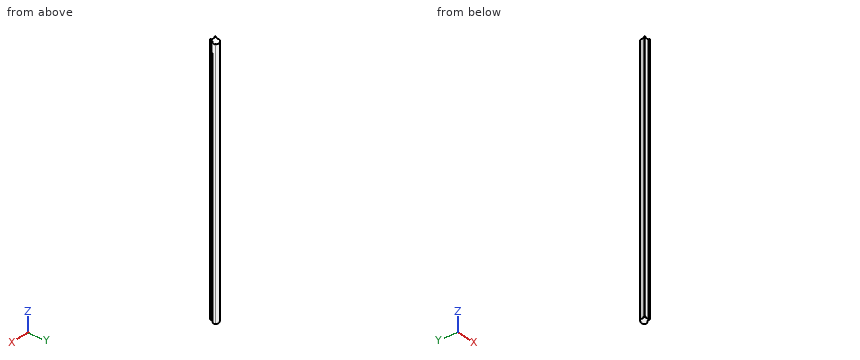
Autodesk Inventor part; units mm, degrees
ref_plane "Конечная плоскость" through (0, 0, 1340.1098) normal (0, 0, 1) x (1, 0, 0)
ref_plane "РабПлоскость4" through (178.641, -785.005, 1769.9053) normal (0, 0.4802388, 0.8771378) x (1, 0, 0)
ref_plane "РабПлоскость5" through (88.641, -691.7426, -766.7409) normal (0, -0.4802388, -0.8771378) x (1, 0, 0)
sketch "Поручень" plane through (0, 0, 0) normal (0, 0, 1) x (1, 0, 0)
  line L0 (20.3655, -7.6059) -> (20.3655, -0.2092)
  line L1 (20.3655, -0.2092) -> (-19.6345, -0.2092)
  line L2 (-19.6345, -0.2092) -> (-19.6345, -7.6059)
  line L3 (-19.6345, -7.6059) -> (-30.865, -7.6059)
  line L4 (-30.865, -7.6059) -> (-30.865, -5.9622)
  line L5 (-30.865, -5.9622) -> (-32.5087, -5.9622)
  line L6 (-32.5087, -5.9622) -> (-32.5087, 0.6126)
  arc A0 (-30.367, 4.2203) -> (-32.5087, 0.6126) centre (-28.3995, 0.6126) ccw
  arc A1 (-30.367, 4.2203) -> (-30.2973, 18.6123) centre (-34.302, 11.4355) ccw
  arc A2 (-24.2902, 41.7054) -> (-30.2973, 18.6123) centre (-24.2902, 29.3776) ccw
  line L7 (-24.2902, 41.7054) -> (-24.2902, 42.9382)
  arc A3 (25.0211, 42.9382) -> (-24.2902, 42.9382) centre (0.3655, 2.9211) ccw
  line L8 (25.0211, 42.9382) -> (25.0211, 41.7054)
  arc A4 (31.0282, 18.6123) -> (25.0211, 41.7054) centre (25.0211, 29.3776) ccw
  arc A5 (31.0282, 18.6123) -> (31.0979, 4.2203) centre (35.033, 11.4355) ccw
  arc A6 (33.2397, 0.6126) -> (31.0979, 4.2203) centre (29.1304, 0.6126) ccw
  line L9 (33.2397, 0.6126) -> (33.2397, -5.9622)
  line L10 (33.2397, -5.9622) -> (31.596, -5.9622)
  line L11 (31.596, -5.9622) -> (31.596, -7.6059)
  line L12 (31.596, -7.6059) -> (20.3655, -7.6059)
  point P0 (0.3655, -0.2092)
  point P1 (0.3655, -7.6059)
sketch "Эскиз" plane through (0, 0, 0) normal (0, 0, 1) x (1, 0, 0)
  line L0 (20, 0) -> (20, 7.3967)
  line L1 (20, 7.3967) -> (-20, 7.3967)
  line L2 (-20, 7.3967) -> (-20, 0)
  line L3 (-20, 0) -> (-31.2305, 0)
  line L4 (-31.2305, 0) -> (-31.2305, 1.6437)
  line L5 (-31.2305, 1.6437) -> (-32.8742, 1.6437)
  line L6 (-32.8742, 1.6437) -> (-32.8742, 8.2186)
  arc A0 (-30.7325, 11.8262) -> (-32.8742, 8.2186) centre (-28.7649, 8.2186) ccw
  arc A1 (-30.7325, 11.8262) -> (-30.6628, 26.2183) centre (-34.6675, 19.0415) ccw
  arc A2 (-24.6557, 49.3113) -> (-30.6628, 26.2183) centre (-24.6557, 36.9835) ccw
  line L7 (-24.6557, 49.3113) -> (-24.6557, 50.5441)
  arc A3 (24.6557, 50.5441) -> (-24.6557, 50.5441) centre (0, 10.527) ccw
  line L8 (24.6557, 50.5441) -> (24.6557, 49.3113)
  arc A4 (30.6628, 26.2183) -> (24.6557, 49.3113) centre (24.6557, 36.9835) ccw
  arc A5 (30.6628, 26.2183) -> (30.7325, 11.8262) centre (34.6675, 19.0415) ccw
  arc A6 (32.8742, 8.2186) -> (30.7325, 11.8262) centre (28.7649, 8.2186) ccw
  line L9 (32.8742, 8.2186) -> (32.8742, 1.6437)
  line L10 (32.8742, 1.6437) -> (31.2305, 1.6437)
  line L11 (31.2305, 1.6437) -> (31.2305, 0)
  line L12 (31.2305, 0) -> (20, 0)
  point P0 (0, 0)
ref_plane "Начальная плоскость" through (0, 0, -1176.9727) normal (0, 0, 1) x (1, 0, 0)
ref_plane "РабПлоскость2" through (0, 0, 1691.8665) normal (0, 0, 1) x (1, 0, 0)
extrude "Тело" add sketch "Эскиз" along normal up to surface (2517.0825 mm away) from surface at -1176.9727
ref_plane "Конечная плоскость" through (0, 0, 1340.1098) normal (0, 0, 1) x (1, 0, 0)
ref_plane "РабПлоскость4" through (178.641, -785.005, 1769.9053) normal (0, 0.4802388, 0.8771378) x (1, 0, 0)
split "Разделение1" plane through (178.641, -785.005, 1769.9053) removes the side toward (0, 0.4802388, 0.8771378)
ref_plane "РабПлоскость5" through (88.641, -691.7426, -766.7409) normal (0, -0.4802388, -0.8771378) x (1, 0, 0)
split "Разделение2" plane through (88.641, -691.7426, -766.7409) removes the side toward (0, -0.4802388, -0.8771378)
equation "\"ШИРИНА\" = 75"
equation "\"ТОЛЩВЫС\" = 58"
equation "\"d0\" = -G_OFFSET_START"
equation "\"СЕЧЕНИЕ_СМЕЩ\" = 0"
equation "\"G_OFFSET_END\" = -351.75672"
equation "\"d4\" = ДЛИНА + G_OFFSET_END"
equation "\"G_OFFSET_START\" = 1176.97268"
equation "\"G_L\" = ДЛИНА + G_OFFSET_START + G_OFFSET_END"
properties part number "Поручень" material "Древесина (дуб)"
CAD build for the part. Positions are in the model's coordinates, mm. Round coordinates to 2 decimals unless told otherwise and drop trailing zeros. Loops run counter-clockwise (first coordinate to the right, second up) from the corner with the lowest first, then second, coordinate; pieces in that order, holes last. Notation, with made-up numbers: M 71,-25 L 78,-25 A18 cw 78,-8 Z; hole C 85,-20 d8. An arc over 180 degrees is marked long. Use a Markdown table: item, result. Add a question column.
(1) Cut at B-B (x = -7). Give the cut face in (y, z), and give its area (3 significant figures).
(2) Cut at A-A (z = 447.5). Give the cut face in (x, y), and give its area (3 significant figures).
(3) Drill centre lines: line 1 (X direction, y = 6.5, z = 1048); line 2 (X direction, y = 40, z = 938); line 3 (Y direction, x = -2.5, z = -538.5). Where is each one in solid material? Low to high.
(4) Flat gauge pins, fed straight in: pin 1 (1.3 mm diameter, centred on y = 0.5, z = -268, fed in from +X); pin 2 (3 mm diameter, centred on x = -26, y = 9.5, fed in from -Z); pin 3 (1.8 mm diameter, centred on y = 0.5, z = -466, fed in from -X); pin 4 (12 mm diameter, centred on y = 35, z = 646, fed in from +X). Where does each tip first touch, or does it go through?
Geometry says:
| question | item | result |
|---|---|---|
| 1 | outline | M 7.4,-1149.52 L 57.01,-1176.69 L 57.01,1308.9 L 7.4,1336.06 Z |
| 1 | area | 123,000 mm² |
| 2 | outline | M -32.87,1.64 L -31.23,1.64 L -31.23,0 L -20,0 L -20,7.4 L 20,7.4 L 20,0 L 31.23,0 L 31.23,1.64 L 32.87,1.64 L 32.87,8.22 A4.11 ccw 30.73,11.83 A8.22 cw 30.66,26.22 A12.33 ccw 24.66,49.31 L 24.66,50.54 A47 ccw -24.66,50.54 L -24.66,49.31 A12.33 ccw -30.66,26.22 A8.22 cw -30.73,11.83 A4.11 ccw -32.87,8.22 Z |
| 2 | area | 3,170 mm² |
| 3 | line 1 | x = -32.87 to -20, 20 to 32.87 |
| 3 | line 2 | x = -36.61 to 36.61 |
| 3 | line 3 | y = 7.4 to 57.46 |
| 4 | pin 1 | stops at x = 31.23 |
| 4 | pin 2 | stops at z = -1151.5 |
| 4 | pin 3 | stops at x = -31.23 |
| 4 | pin 4 | stops at x = 36.98 |
